Read the model definition and answer for the solid it produces. Units are mm, in the model's axes. A direction names the side the tool comes from. Round coordinates to 2 decimals unless told otherwise and drop trailing zeros. Loops run counter-clockwise (first coordinate to the right, second up) from the corner with the lowest first, then second, coordinate; pieces in that order, holes last. Notation, with made-up numbers: (61, -27) - (107, -27) arc R26 cw to (107, 5) - close; hole circle Ø7 at (-26, -32.75). An arc over 180 degrees is marked (long way). Use CSV: the item, a comma, the result in double quotes. Start each with the question number.
1. Given pin 1 Ø4 at (x, y) = (-7.5, 67.5) entering from +Z; pin 2 Ø2.5 at (x, z) = (-12.7, 29.95) entering from +Y, each flat-ended and moving along its own axis, determine where each tip first touches the part or whether it passes through.
2. A tool of negligible diameter and unlimited length cuts with its end or side. For faces 3 (the flat face through (0, 108.648, 19)), 4 (the flat face through (0, 1, 0)), from which of +Z, -Z, +X, -X, +Y, -Y can it reach the whole face along a straight path? Write none if from no direction.
3. Find section A-A (z = 24). Give the vertices of the cut face in (x, y), and give its area (3 significant figures).
4. Determine the mould class of faces 1 (the flat face through (0, 1, -0.889)), 2 (the cylindrical face through (-5.03, 108.21, 10.02)) for opening direction X: +X half, -X half, draft (parallel to the pull), parting line (faces both ways), or undercut.
5. Consider line 1 along Y through (x, z) = (-17, 32.5); line 2 along Z through (x, y) = (-3.81, -107.95); line 3 along Z through (x, y) = (15.5, -61). Determine where each line is inside the solid, lowest interval first.
6. Find section D-D (y = -6). Give the vertices of the cut face in (x, z).
7. Find section C-C (x = 13). Give the vertices of the cut face in (y, z), and give its area (3 significant figures).
8. Find section B-B (x = -3.81). Give the vertices of the cut face in (y, z).
from build123d import *

# Parameters (mm, degrees)
SKETCH1_W                        = 38.1
SKETCH1_H                        = 292.1
BASE_FLANGE1_DEPTH               = 0.889
SKETCHED_START                   = -19.05
SKETCHED_BEND5_DEPTH             = 38.1
SKETCHED_BEND5_2_DEPTH           = 38.1
SKETCHED_BEND8_DEPTH             = 38.1
SKETCHED_BEND8_2_DEPTH           = 38.1
F_1_4_0_25_DIAMETER_HOLE4_D      = 6.35
F_1_4_0_25_DIAMETER_HOLE4_DEPTH  = 0.889
F_1_8_0_125_DIAMETER_HOLE1_D     = 3.175
F_1_8_0_125_DIAMETER_HOLE1_DEPTH = 0.889


# Read off the part's stored shape, not the designer's step: Sketched Bend5, Sketched Bend8
# Sheet-metal steps are written as plain solids
with BuildPart() as part:
    # Sketch1 → Base-Flange1 (new body)
    with BuildSketch(Plane.XY):
        Rectangle(SKETCH1_W, SKETCH1_H)
    extrude(amount=-BASE_FLANGE1_DEPTH)

    # Sketched Bend5 outline → Sketched Bend5 (cut)
    with BuildSketch(Plane.YZ.offset(SKETCHED_START)):
        with BuildLine():
            Line((146.05, 0), (108.471502454, 0))
            ThreePointArc((108.471502454, 0), (107.872412816, -0.64903926), (107.022366229, -0.889))
            Line((107.022366229, -0.889), (146.05, -0.889))
            Line((146.05, -0.889), (146.05, 0))
        make_face()
    extrude(amount=SKETCHED_BEND5_DEPTH, mode=Mode.SUBTRACT)

    # Sketched Bend5 2 outline → Sketched Bend5 2 (add)
    with BuildSketch(Plane.YZ.offset(SKETCHED_START)):
        with BuildLine():
            ThreePointArc((108.471502454, 0), (108.603234852, 0.357878789), (108.647966229, 0.7366))
            Line((108.647966229, 0.7366), (108.647966229, 37.908966229))
            Line((108.647966229, 37.908966229), (107.758966229, 37.908966229))
            Line((107.758966229, 37.908966229), (107.758966229, 0.7366))
            ThreePointArc((107.758966229, 0.7366), (107.543221084, 0.215745145), (107.022366229, 0))
            Line((107.022366229, 0), (108.471502454, 0))
        make_face()
    extrude(amount=SKETCHED_BEND5_2_DEPTH)

    # Sketched Bend8 outline → Sketched Bend8 (cut)
    with BuildSketch(Plane.YZ.offset(SKETCHED_START)):
        with BuildLine():
            ThreePointArc((-107.022366229, -0.889), (-107.872412816, -0.64903926), (-108.471502454, 0))
            Line((-108.471502454, 0), (-146.05, 0))
            Line((-146.05, 0), (-146.05, -0.889))
            Line((-146.05, -0.889), (-107.022366229, -0.889))
        make_face()
    extrude(amount=SKETCHED_BEND8_DEPTH, mode=Mode.SUBTRACT)

    # Sketched Bend8 2 outline → Sketched Bend8 2 (add)
    with BuildSketch(Plane.YZ.offset(SKETCHED_START)):
        with BuildLine():
            Line((-107.758966229, 0.7366), (-107.758966229, 37.908966229))
            Line((-107.758966229, 37.908966229), (-108.647966229, 37.908966229))
            Line((-108.647966229, 37.908966229), (-108.647966229, 0.7366))
            ThreePointArc((-108.647966229, 0.7366), (-108.603234852, 0.357878789), (-108.471502454, 0))
            Line((-108.471502454, 0), (-107.022366229, 0))
            ThreePointArc((-107.022366229, 0), (-107.543221084, 0.215745145), (-107.758966229, 0.7366))
        make_face()
    extrude(amount=SKETCHED_BEND8_2_DEPTH)

    # 1/4 (0.25) Diameter Hole4
    with Locations(Plane(origin=(-3.81, 107.758966229, 7.0866), x_dir=(0, 0, -1), z_dir=(0, -1, 0))):
        with Locations((0, 0)):
            f_1_4_0_25_diameter_hole4 = Hole(F_1_4_0_25_DIAMETER_HOLE4_D / 2, depth=F_1_4_0_25_DIAMETER_HOLE4_DEPTH)

    # 1/8 (0.125) Diameter Hole1
    with Locations(Plane(origin=(-12.7, 107.758966229, 29.9466), x_dir=(0, 0, -1), z_dir=(0, -1, 0))):
        with Locations((0, 0)):
            f_1_8_0_125_diameter_hole1 = Hole(F_1_8_0_125_DIAMETER_HOLE1_D / 2, depth=F_1_8_0_125_DIAMETER_HOLE1_DEPTH)

    # Mirror1: 1/4 (0.25) Diameter Hole4, 1/8 (0.125) Diameter Hole1 across plane
    add(f_1_4_0_25_diameter_hole4.mirror(Plane.ZX), mode=Mode.SUBTRACT)
    add(f_1_8_0_125_diameter_hole1.mirror(Plane.ZX), mode=Mode.SUBTRACT)


solid = part.part
Filled sheet:
1,pin 1,"stops at z = 0"
1,pin 2,"passes through"
2,face 3,"+Z, -Z, +X, -X, +Y"
2,face 4,"+Z, +X, -X"
3,outline,"(-19.05, -108.65) - (19.05, -108.65) - (19.05, -107.76) - (-19.05, -107.76) - close; (-19.05, 107.76) - (19.05, 107.76) - (19.05, 108.65) - (-19.05, 108.65) - close"
3,area,"67.7 mm²"
4,face 1,"draft"
4,face 2,"undercut"
5,line 1,"y = -108.65 to -107.76, 107.76 to 108.65"
5,line 2,"z = -0.6 to 3.91, 10.26 to 37.91"
5,line 3,"z = -0.89 to 0"
6,outline,"(-19.05, -0.89) - (19.05, -0.89) - (19.05, 0) - (-19.05, 0) - close"
7,outline,"(-108.65, 0.74) arc R1.63 ccw to (-107.02, -0.89) - (107.02, -0.89) arc R1.63 ccw to (108.65, 0.74) - (108.65, 37.91) - (107.76, 37.91) - (107.76, 0.74) arc R0.74 cw to (107.02, 0) - (-107.02, 0) arc R0.74 cw to (-107.76, 0.74) - (-107.76, 37.91) - (-108.65, 37.91) - close"
7,area,"260 mm²"
8,outline,"(-108.65, 0.74) arc R1.63 ccw to (-107.02, -0.89) - (107.02, -0.89) arc R1.63 ccw to (108.65, 0.74) - (108.65, 3.91) - (107.76, 3.91) - (107.76, 0.74) arc R0.74 cw to (107.02, 0) - (-107.02, 0) arc R0.74 cw to (-107.76, 0.74) - (-107.76, 3.91) - (-108.65, 3.91) - close; (-108.65, 10.26) - (-107.76, 10.26) - (-107.76, 37.91) - (-108.65, 37.91) - close; (107.76, 10.26) - (108.65, 10.26) - (108.65, 37.91) - (107.76, 37.91) - close"
